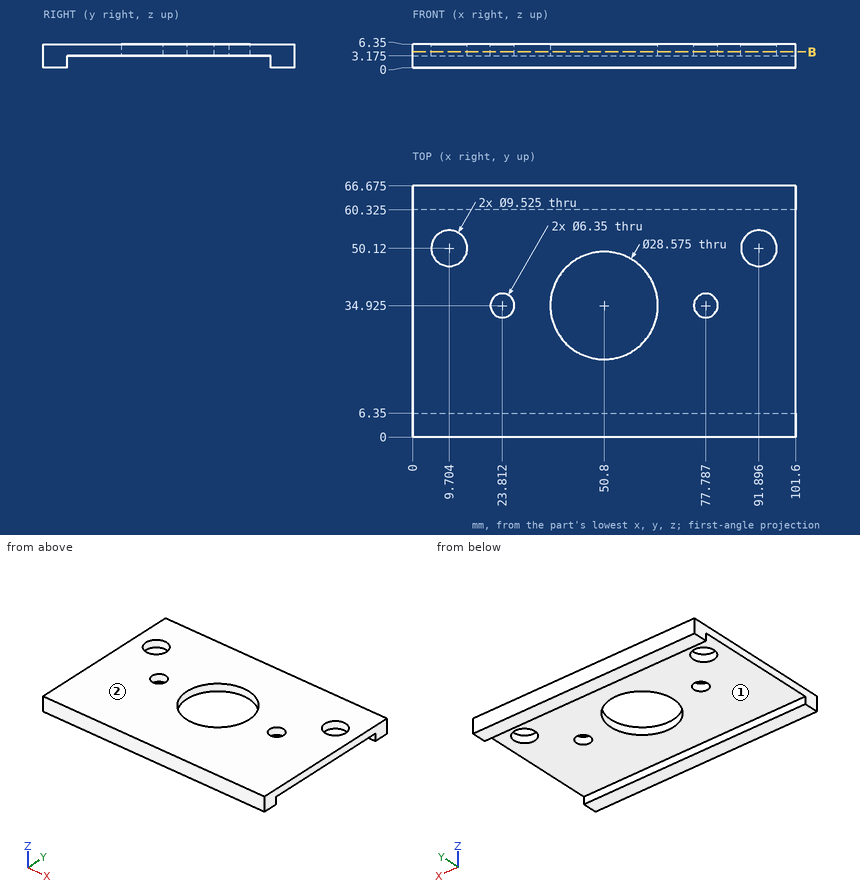
Geometry check sheet. Reference: drawing and pictorial views, mm from the part's lowest x, y, z. A direction names the side the tool comes from. Give positions to 0.01 mm unless a question says otherwise; leave off trailing zeros.
Item 1: Scan lines: L1, parallel to X at y = 51.5, z = 6 (1 decimal); L2, parallel to X at y = 42, z = 3.5; L3, parallel to X at y = 47, z = 6.25 (1 decimal). Record each from-to range of solid material in increasing order.
Item 2: Gauge pin test, flat ends, axial feed: pin 1 (16 mm diameter, centred on x = 47, y = 24, fed in from -Z) (1 decimal); pin 2 (5.5 mm diameter, centred on x = 23.81, y = 34.92, fed in from +Z). Record the tip position at first contact, or that the pin passes through.
Item 3: Cross-section at B-B (z = 4.25). Count the separate pieces of the cut face and the enclosed holes in it, and give its area (3 significant figures).
Item 4: Access from +Z, -Z, +X, -X, +Y, -Y to the whole of each face (thin tool, end or side, straight path). Record for the marked faces 1 and 2.
Report:
1. L1: x = 0 to 5.1, 14.3 to 87.3, 96.5 to 101.6
1. L2: x = 0 to 38.39, 63.21 to 101.6
1. L3: x = 0 to 6.1, 13.3 to 43.2, 58.4 to 88.3, 95.5 to 101.6
2. pin 1: stops at z = 3.2
2. pin 2: passes through
3. separate pieces: 1
3. enclosed holes: 5
3. area: 5,930 mm2
4. face 1: -Z, +X, -X
4. face 2: +Z, +X, -X, +Y, -Y
